The figure shows three views and two pictorial views of one solid part (mm, origin at its lowest corner). Answer the questions. A direction names the side the tool comes from. Round coordinates to 2 decimals unless told otherwise and drop trailing zeros. Order: outer loops, then holes, each group sorted by start corner. A loop starts at its lowest first (then second) coordinate and runs counter-clockwise, first axis right, second up. Notation, with made-up numbers: M 66,-38.75 L 116,-38.75 A25 cw 116,-3.75 Z; hole C 69.5,69.5 d3. An arc over 180 degrees is marked long. Return JSON: item names as keys, results as strings.
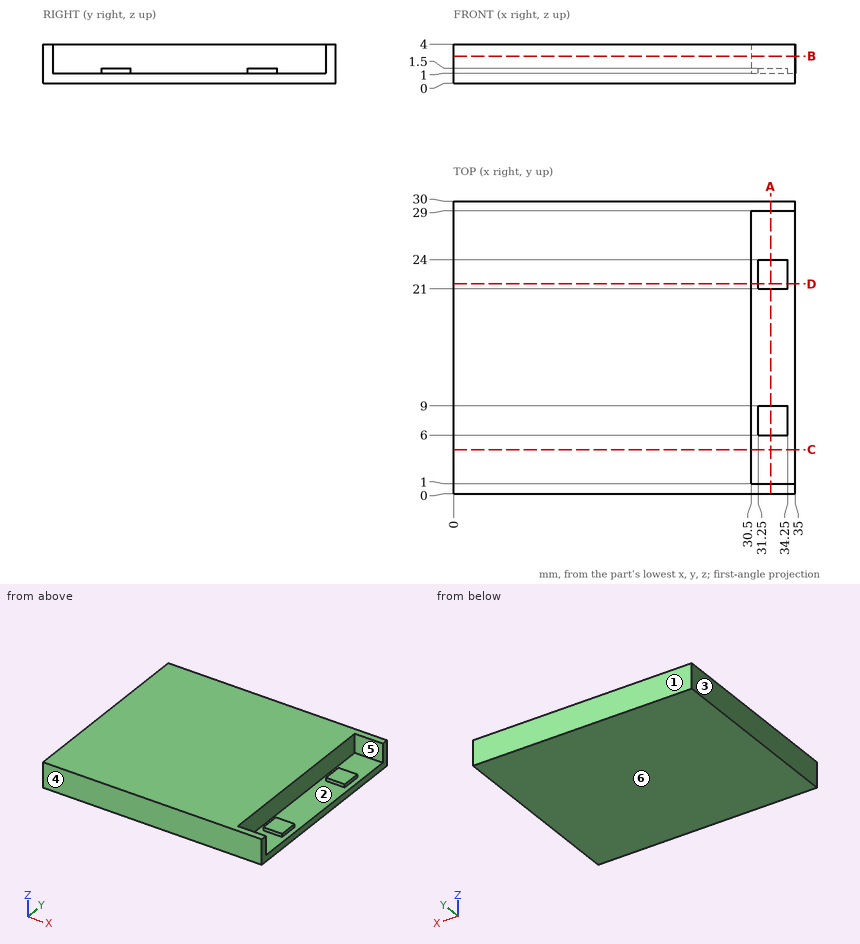
Item 1: Find section D-D (y = 21.5). Determine the outline of the cut face in (x, z), plus the area to 3 significant figures.
Output:
{"outline": "M 0,0 L 35,0 L 35,1 L 34.25,1 L 34.25,1.5 L 31.25,1.5 L 31.25,1 L 30.5,1 L 30.5,4 L 0,4 Z", "area": "128 mm^2"}
Item 2: Find section B-B (z = 2.75). Determine the outline of the cut face in (x, y), plus the area to 3 significant figures.
Output:
{"outline": "M 0,0 L 35,0 L 35,1 L 30.5,1 L 30.5,29 L 35,29 L 35,30 L 0,30 Z", "area": "924 mm^2"}
Item 3: Which of the six approach directions +Z, -Z, +X, -X, +Y, -Y give full straight-line access (tool end or side, diameter ignored) to the marked faces 5 and 6?
Output:
{"face 5": "+Z, +X", "face 6": "-Z, +X, -X, +Y, -Y"}
Item 4: Find section A-A (x = 32.5). Determine the outline of the cut face in (y, z), plus the area to 3 significant figures.
Output:
{"outline": "M 0,0 L 30,0 L 30,4 L 29,4 L 29,1 L 24,1 L 24,1.5 L 21,1.5 L 21,1 L 9,1 L 9,1.5 L 6,1.5 L 6,1 L 1,1 L 1,4 L 0,4 Z", "area": "39.0 mm^2"}
Item 5: The mould has two halves that part along Y. Classify the marked faces 1, 2, 3 and 4: pulls with the +Y half, pulls with the -Y half, needs draft (parallel to the pull), parting line crosses it, or undercut.
Output:
{"face 1": "pulls with the +Y half", "face 2": "undercut", "face 3": "needs draft", "face 4": "pulls with the -Y half"}
Item 6: Consider line 1 along X through (y, z) = (10.75, 2.4); line 2 along Z through (x, y) = (31, 21). Determine where each line is inside the solid, lowest interval first. Write a range as [from, to].
Output:
{"line 1": "x = [0, 30.5]", "line 2": "z = [0, 1]"}
Item 7: Find section C-C (y = 4.5). Determine the outline of the cut face in (x, z).
Output:
{"outline": "M 0,0 L 35,0 L 35,1 L 30.5,1 L 30.5,4 L 0,4 Z"}
Item 8: Each of these flat-tipped pins is pushed along its axis until it touches: pin 1 (1.5 mm diameter, centred on y = 16.5, z = 2.5, fed in from +X); pin 2 (0.9 mm diameter, centred on x = 32.5, y = 8, fed in from +Z). Where does it stop, or does it pass through?
Output:
{"pin 1": "stops at x = 30.5", "pin 2": "stops at z = 1.5"}
